Autodesk Inventor part; units mm, degrees
ref_plane "YZ Plane" through (0, 0, 0) normal (1, 0, 0) x (0, 1, 0)
ref_plane "XZ Plane" through (0, 0, 0) normal (0, 1, 0) x (-1, 0, 0)
ref_plane "XY Plane" through (0, 0, 0) normal (0, 0, 1) x (1, 0, 0)
sketch "Sketch1" plane through (0, 0, 0) normal (0, 0, 1) x (1, 0, 0)
  line L0 (-110, -50) -> (110, -50)
  line L1 (110, -50) -> (110, 50)
  line L2 (110, 50) -> (-110, 50)
  line L3 (-110, 50) -> (-110, -50)
  line L4 (-110, -50) -> (110, 50) construction
  circle A0 centre (-62.5, 0) radius 7.5
  circle A1 centre (62.5, 0) radius 7.5
  line L5 (0, 50) -> (0, -50) construction
  line L6 (-110, 0) -> (110, 0) construction
  line L7 (-70, 0) -> (-55, 0) construction
  point P0 (0, 0)
  dimension "d154" = 220
  dimension "d155" = 100
  dimension "d159" = 15
  dimension "d160" = 125
  dimension "d190" = 15
extrude "Plate5" add sketch "Sketch1" along normal blind 3
sketch "Sketch7" plane through (-107, 50, 3) normal (-1, 0, 0) x (0, -1, 0)
  line L0 (100, 0) -> (0, 0)
  line L1 (0, 0) -> (0, -90)
  line L2 (0, -90) -> (100, -90)
  line L3 (100, -90) -> (100, 0)
edge flange "Flange3" height 90 angle 90 thickness 3 bend radius 3 thickness toward (-1, 0, 0) relief tear relief width 3 relief depth 1.5 corner gap 3 corner form 0 edges at (-110, 0, 0) (110, 0, 0) wall of the first edge with corners at (-107, -50, 3) (-107, 50, 3) (-107, 50, -87) (-107, -50, -87)
bend "Bend3"
corner "Corner3"
sketch "Sketch8" plane through (-107, -50, -84) normal (0, 0, -1) x (-1, 0, 0)
  line L0 (0, 100) -> (0, 0)
  line L1 (0, 0) -> (35, 0)
  line L2 (35, 0) -> (35, 100)
  line L3 (35, 100) -> (0, 100)
edge flange "Flange4" height 35 angle 90 thickness 3 bend radius 3 thickness toward (0, 0, -1) relief tear relief width 3 relief depth 1.5 corner gap 3 corner form 0 edges at (-110, 0, -87) (110, 0, -87) wall of the first edge with corners at (-107, 50, -84) (-107, -50, -84) (-142, -50, -84) (-142, 50, -84)
bend "Bend4"
corner "Corner4"
sketch "Sketch9" plane through (-142, -50, -87) normal (0, 0, -1) x (-1, 0, 0)
  line L0 (-10.5, 9.5) -> (-10.5, 24.5) construction
  line L1 (-5, 9.5) -> (-5, 24.5)
  line L2 (-16, 24.5) -> (-16, 9.5)
  arc A0 (-16, 9.5) -> (-5, 9.5) centre (-10.5, 9.5) ccw
  arc A1 (-5, 24.5) -> (-16, 24.5) centre (-10.5, 24.5) ccw
  line L3 (-10.5, 75.5) -> (-10.5, 90.5) construction
  line L4 (-5, 75.5) -> (-5, 90.5)
  line L5 (-16, 90.5) -> (-16, 75.5)
  arc A2 (-16, 75.5) -> (-5, 75.5) centre (-10.5, 75.5) ccw
  arc A3 (-5, 90.5) -> (-16, 90.5) centre (-10.5, 90.5) ccw
  line L6 (0, 100) -> (0, 0)
  line L7 (0, 50) -> (-19.5858, 50)
  point P0 (-142, 50)
  point P1 (-10.5, 17)
  point P2 (-10.5, 83)
  point P3 (-10.5, 30)
  point P4 (-10.5, 70)
  dimension "d182" = 11
  dimension "d183" = 15
  dimension "d184" = 5
  dimension "d186" = 40
extrude "Cut1" cut sketch "Sketch9" against normal blind 3
mirror "Mirror1" about plane through (0, 0, 0) normal (1, 0, 0) of "Cut1"
fillet "Corner Round2" radius 2 4 edges at (-142, 50, -85.5) (-142, -50, -85.5) (142, -50, -85.5) (142, 50, -85.5)
properties part number "DMF Подставка ркдуктор_CPY"
The model under review builds one solid part; all positions refer to its coordinate system, in mm. A direction names the side the tool comes from. Round coordinates to 2 decimals unless told otherwise and drop trailing zeros. Loops run counter-clockwise (first coordinate to the right, second up) from the corner with the lowest first, then second, coordinate; pieces in that order, holes last. Notation, with made-up numbers: M 0,-3 L 40,-3 A15 ccw 40,16 Z; hole C -10.5,68.5 d8. An arc over 180 degrees is marked long. Answer as CSV lines item,"result". Start each with the question number.
Item 1: Consider section A-A (z = -27). Write out the cut boundary in (x, y), then the cut area to 3 significant figures.
Item 2: Wall thickness on line 1 (X direction, y = 16.5, z = -20); line 2 (Y direction, x = 62, z = 1); line 3 (Z direction, x = 113, y = 21.5): over which ranges is each line inside the solid? List them lowest first. Write a range as [from, to].
Item 3: Consider section C-C (x = -131.5). Write out the cut boundary in (y, z).
Item 4: Consider section B-B (y = 0). Write out the cut boundary in (x, z), then the cut area to 3 significant figures.
Item 5: Consider section D-D (y = 12). Write out the cut boundary in (x, z).
Item 6: Insertion check: P1, Ø1, axis at y = 12.5, z = -61, coming from the -X side; P2, Ø5, axis at y = -34.5, z = -64, coming from the +X side; P3, Ø12, axis at x = 62.5, y = 0, coming from the -Z side; P4, Ø14.5, axis at x = 128.5, y = 4, coming from the +Z side. Each pin has a flat end and moves straight along its axis. Give the tip position at first contact, or say it passes through.
Item 7: For faces 5 (the face through (-108.804, -0.7, -85.289)), 6 (the face through (110, -1, -43)), 7 (the face through (131.6, 20, -85.5)), 8 (the face through (-110, 1, -43)), list the 3-axis set-ups (+Z, -Z, +X, -X, +Y, -Y) from which the entire face can be reached by the end or side of a thin tool; tool diameter is ignored.
Item 8: Mouldability with a two-part tool opening along X and no side actions: class faces 1 (the face through (-1, 1, 0)), 2 (the face through (128, 1, -87)), 3 (the face through (131.6, -46, -85.5)), 4 (the face through (-108.289, 0.7, 1.196)) as released by +X, released by -X, zero draft, split by the parting line, or undercut.
Answer:
1,outline,"M -110,-50 L -107,-50 L -107,50 L -110,50 Z; M 107,-50 L 110,-50 L 110,50 L 107,50 Z"
1,area,"600 mm^2"
2,line 1,"x = [-110, -107], [107, 110]"
2,line 2,"y = [-50, -7.48], [7.48, 50]"
2,line 3,"z = [-87, -84]"
3,outline,"M -50,-87 L -46,-87 L -46,-84 L -50,-84 Z; M -20,-87 L 20,-87 L 20,-84 L -20,-84 Z; M 46,-87 L 50,-87 L 50,-84 L 46,-84 Z"
4,outline,"M -142,-87 L -113,-87 A6 ccw -107,-81 L -107,-3 A3 cw -104,0 L -70,0 L -70,3 L -104,3 A6 ccw -110,-3 L -110,-81 A3 cw -113,-84 L -142,-84 Z; M -55,0 L 55,0 L 55,3 L -55,3 Z; M 70,0 L 104,0 A3 cw 107,-3 L 107,-81 A6 ccw 113,-87 L 142,-87 L 142,-84 L 113,-84 A3 cw 110,-81 L 110,-3 A6 ccw 104,3 L 70,3 Z"
4,area,"1,260 mm^2"
5,outline,"M -142,-87 L -113,-87 A6 ccw -107,-81 L -107,-3 A3 cw -104,0 L 104,0 A3 cw 107,-3 L 107,-81 A6 ccw 113,-87 L 142,-87 L 142,-84 L 113,-84 A3 cw 110,-81 L 110,-3 A6 ccw 104,3 L -104,3 A6 ccw -110,-3 L -110,-81 A3 cw -113,-84 L -142,-84 Z"
6,P1,"stops at x = -110"
6,P2,"stops at x = 110"
6,P3,"passes through"
6,P4,"stops at z = -84"
7,face 5,"-Z, +Y, -Y"
7,face 6,"+Z, +X, +Y, -Y"
7,face 7,"+Z, -Z"
7,face 8,"+Z, -X, +Y, -Y"
8,face 1,"undercut"
8,face 2,"zero draft"
8,face 3,"undercut"
8,face 4,"released by -X"
